from build123d import *

# Parameters (mm, degrees)
SKETCH1_W           = 17.28
SKETCH1_H           = 18.2
BOSS_EXTRUDE1_DEPTH = 2.6


with BuildPart() as part:
    # Sketch1 → Boss-Extrude1 (new body, symmetric)
    with BuildSketch(Plane.XY):
        Polygon((-0.1, 66.95), (-0.1, 44.55), (-0.1, 39.4), (-0.1, 27.45), (-0.1, 22.3), (-0.1, -0.1), (25.1, -0.1), (25.1, 22.3), (25.1, 27.45), (25.1, 39.4), (25.1, 44.55), (25.1, 66.95), align=None)
        with Locations((12.5, 50.525)):
            Rectangle(SKETCH1_W, SKETCH1_H, mode=Mode.SUBTRACT)
    extrude(amount=BOSS_EXTRUDE1_DEPTH, both=True)


solid = part.part
The model under review builds one solid part; all positions refer to its coordinate system, in mm. A direction names the side the tool comes from. Coordinates: 2 decimals unless noted, no trailing zeros. Loops run counter-clockwise (first coordinate to the right, second up) from the corner with the lowest first, then second, coordinate; pieces in that order, holes last.
(1) Consider section A-A, the plane y = 54. Give the boundary of the cut face in (x, z), plus the area to 3 significant figures.
Determined:
outline: (-0.1, -2.6) - (3.86, -2.6) - (3.86, 2.6) - (-0.1, 2.6) - close; (21.14, -2.6) - (25.1, -2.6) - (25.1, 2.6) - (21.14, 2.6) - close
area: 41.2 mm2
(2) Wall thickness on L1, parallel to X at y = 54.5, z = -2.2; L2, parallel to Y at x = 14.75, z = 0.45 (3 decimals): over which ranges is each line inside the solid? List them lowest first.
Determined:
L1: x = -0.1 to 3.86, 21.14 to 25.1
L2: y = -0.1 to 41.425, 59.625 to 66.95
(3) Tool access review of faces 1 (the flat face through (21.14, 50, 0)), 2 (the flat face through (25.1, 33, 0)): name each direction out of +Z, -Z, +X, -X, +Y, -Y from which nothing blocks a thin tool from reaching the whole face with its end or side.
Determined:
face 1: +Z, -Z
face 2: +Z, -Z, +X, +Y, -Y
(4) Consider section C-C, the plane z = -2. Give the boundary of the cut face in (x, y) (3 decimals), plus the area to 3 significant figures.
Determined:
outline: (-0.1, -0.1) - (25.1, -0.1) - (25.1, 66.95) - (-0.1, 66.95) - close; hole (3.86, 41.425) - (21.14, 41.425) - (21.14, 59.625) - (3.86, 59.625) - close
area: 1,380 mm2
(5) Draft analysis for pull direction X (two halves, no side actions). For faces 3 (the flat face through (12, 26, -2.6)), 4 (the flat face through (3.86, 50, 0)), 5 (the flat face through (-0.1, 34, 0)), state which applies: +X half, -X half, draft (parallel to the pull), parting line (faces both ways), or undercut.
Determined:
face 3: draft
face 4: undercut
face 5: -X half
(6) Consider section B-B, the plane x = 11.5. Give the boundary of the cut face in (y, z) (3 decimals), plus the area to 3 significant figures.
Determined:
outline: (-0.1, -2.6) - (41.425, -2.6) - (41.425, 2.6) - (-0.1, 2.6) - close; (59.625, -2.6) - (66.95, -2.6) - (66.95, 2.6) - (59.625, 2.6) - close
area: 254 mm2
